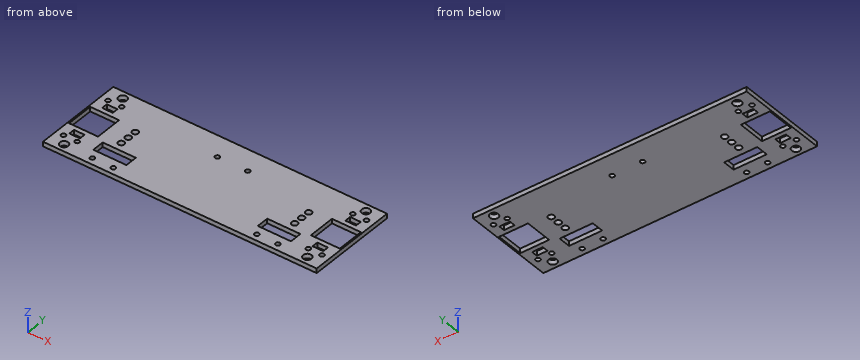
from build123d import *

# Parameters (mm, degrees)
SKETCH_W   = 90
SKETCH_H   = 60
SKETCH_R   = 2.75
SKETCH_R_2 = 2
SKETCH_R_3 = 1.5
SKETCH_W_2 = 7
SKETCH_H_2 = 4
SKETCH_W_3 = 19
SKETCH_H_3 = 18
SKETCH_W_4 = 21.8
SKETCH_H_4 = 8
PAD_DEPTH  = 3


with BuildPart() as part:
    # Sketch → Pad (new body)
    with BuildSketch(Plane.XY):
        with Locations((45, 30)):
            Rectangle(SKETCH_W, SKETCH_H)
        with Locations((10, 5)):
            Circle(SKETCH_R, mode=Mode.SUBTRACT)
        with Locations((33, 24)):
            Circle(SKETCH_R_2, mode=Mode.SUBTRACT)
        with Locations((33, 36)):
            Circle(SKETCH_R_2, mode=Mode.SUBTRACT)
        with Locations((33, 30)):
            Circle(SKETCH_R_2, mode=Mode.SUBTRACT)
        with Locations((10, 55)):
            Circle(SKETCH_R, mode=Mode.SUBTRACT)
        with Locations((14, 11)):
            Circle(SKETCH_R_3, mode=Mode.SUBTRACT)
        with Locations((5, 11)):
            Circle(SKETCH_R_3, mode=Mode.SUBTRACT)
        with Locations((14, 49)):
            Circle(SKETCH_R_3, mode=Mode.SUBTRACT)
        with Locations((5, 49)):
            Circle(SKETCH_R_3, mode=Mode.SUBTRACT)
        with Locations((80, 45)):
            Circle(SKETCH_R_3, mode=Mode.SUBTRACT)
        with Locations((29, 4.5)):
            Circle(SKETCH_R_3, mode=Mode.SUBTRACT)
        with Locations((42.8, 4.5)):
            Circle(SKETCH_R_3, mode=Mode.SUBTRACT)
        with Locations((10, 16)):
            Rectangle(SKETCH_W_2, SKETCH_H_2, mode=Mode.SUBTRACT)
        with Locations((10, 44)):
            Rectangle(SKETCH_W_2, SKETCH_H_2, mode=Mode.SUBTRACT)
        with Locations((10.5, 30)):
            Rectangle(SKETCH_W_3, SKETCH_H_3, mode=Mode.SUBTRACT)
        with Locations((35.9, 14.5)):
            Rectangle(SKETCH_W_4, SKETCH_H_4, mode=Mode.SUBTRACT)
    pad = extrude(amount=PAD_DEPTH)

    # Mirrored: Pad across face of Pad
    add(pad.mirror(Plane(origin=(90, 30, 1.5), x_dir=(0, 1, 0), z_dir=(1, 0, 0))))


solid = part.part
For this review, take the finished solid that the model builds, in its own axes (mm). Give positions to 0.01 mm unless a question says otherwise; leave off trailing zeros. Order: outer loops, then holes, each group sorted by start corner. A loop starts at its lowest first (then second) coordinate and runs counter-clockwise, first axis right, second up. Notation, with made-up numbers: M 39.5,-36 L 82.5,-36 A32 cw 82.5,3 Z; hole C 59.25,48.25 d1. An arc over 180 degrees is marked long. Answer in a Markdown table with one row per item. Add a question column.
(1) Consider section B-B on x = 147. State the section outline as (y, z) points.
(2) Wall thickness on probe 1 along Y at (x, z) = (170, 2.3); probe 2 along Y at (x, z) = (14, 1.45); probe 3 along Y at (x, z) = (140, 1.35): over which ranges is each line inside the solid? List them lowest first. Write a range as [from, to].
(3) Consider section C-C on z = 1.8. Give the number of separate pieces and of enclosed holes in the cut face, and give its area (3 significant figures).
(4) Consider section A-A on x = 170. State the section outline as (y, z) points, and give its area (3 significant figures).
Evaluation:
| question | item | result |
|---|---|---|
| 1 | outline | M 0,0 L 10.5,0 L 10.5,3 L 0,3 Z; M 18.5,0 L 22,0 L 22,3 L 18.5,3 Z; M 26,0 L 28,0 L 28,3 L 26,3 Z; M 32,0 L 34,0 L 34,3 L 32,3 Z; M 38,0 L 60,0 L 60,3 L 38,3 Z |
| 2 | probe 1 | y = [0, 2.25], [7.75, 14], [18, 21], [39, 42], [46, 52.25], [57.75, 60] |
| 2 | probe 2 | y = [0, 9.5], [12.5, 21], [39, 47.5], [50.5, 60] |
| 2 | probe 3 | y = [0, 10.5], [18.5, 60] |
| 3 | separate pieces | 1 |
| 3 | enclosed holes | 32 |
| 3 | area | 9,390 mm^2 |
| 4 | outline | M 0,0 L 2.25,0 L 2.25,3 L 0,3 Z; M 7.75,0 L 14,0 L 14,3 L 7.75,3 Z; M 18,0 L 21,0 L 21,3 L 18,3 Z; M 39,0 L 42,0 L 42,3 L 39,3 Z; M 46,0 L 52.25,0 L 52.25,3 L 46,3 Z; M 57.75,0 L 60,0 L 60,3 L 57.75,3 Z |
| 4 | area | 69.0 mm^2 |
